from build123d import *

# Parameters (mm, degrees)
F1_DEPTH = 127
F2_R     = 242.677577
F3_DEPTH = 25.4
F4_R     = 14.944068
F5_DEPTH = 25.4
F6_DEPTH = 25.4
F7_DEPTH = 127.001


with BuildPart() as f1:
    # F0 (on Front) → F1 (new body)
    with BuildSketch(Plane.XZ):
        with BuildLine():
            Line((-211.768046, 98.819412), (-148.323849, 98.819412))
            Line((-148.323849, 98.819412), (-148.323849, -113.029018))
            ThreePointArc((-148.323849, -113.029018), (-234.634399, -80.514054), (-279.625744, 0))
            ThreePointArc((-279.625744, 0), (-245.041574, -121.948367), (-126.808003, -167.646199))
            ThreePointArc((-126.808003, -167.646199), (-8.574432, -121.948367), (26.009738, 0))
            ThreePointArc((26.009738, 0), (-18.981606, -80.514054), (-105.292156, -113.029018))
            Line((-105.292156, -113.029018), (-105.292156, 98.819412))
            Line((-105.292156, 98.819412), (-37.183784, 98.819412))
            Line((-37.183784, 98.819412), (-37.183784, 140.196055))
            Line((-37.183784, 140.196055), (-103.637077, 140.196055))
            Line((-103.637077, 140.196055), (-103.637077, 178.814262))
            Line((-103.637077, 178.814262), (-148.323849, 178.814262))
            Line((-148.323849, 178.814262), (-148.323849, 140.196055))
            Line((-148.323849, 140.196055), (-211.768046, 140.196055))
            Line((-211.768046, 140.196055), (-211.768046, 98.819412))
        make_face()
    extrude(amount=F1_DEPTH)

    # F2 (on Front) → F3 (join)
    with BuildSketch(Plane.XZ):
        with Locations((-129.646823, -14.895595)):
            Circle(F2_R)
    extrude(amount=F3_DEPTH)

    # F4 (on Front) → F5 (join)
    with BuildSketch(Plane.XZ):
        with Locations((-127.059489, 204.872638)):
            Circle(F4_R)
    extrude(amount=F5_DEPTH)

    # F4 (on Front) → F6 (join)
    with BuildSketch(Plane.XZ):
        with Locations((-127.059489, 204.872638)):
            Circle(F4_R)
    extrude(amount=F6_DEPTH)

    # F4 (on Front) → F7 (cut, through all)
    with BuildSketch(Plane.XZ):
        with Locations((-127.059489, 204.872638)):
            Circle(F4_R)
    extrude(amount=F7_DEPTH, mode=Mode.SUBTRACT)


solid = f1.part
Geometry: final body of the model. Coordinates: model frame, mm. A direction names the side the tool comes from. Round coordinates to 2 decimals unless told otherwise and drop trailing zeros. Loops run counter-clockwise (first coordinate to the right, second up) from the corner with the lowest first, then second, coordinate; pieces in that order, holes last.
Q1. Pin query (flat end, axial travel): P1, Ø1.5, axis at x = -227, y = -83, coming from the +Z side; P2, Ø11.5, axis at y = -58, z = 153, coming from the -X side; P3, Ø6, axis at x = -24.5, y = -92, coming from the -Z side. Return the tip coordinate at first contact, or that it passes through.
Q2. Access query for faces 1 (the flat face through (-126, -75, 178.814)), 2 (the cylindrical face through (-17.99, -75.49, -79.65)), 3 (the flat face through (-211.768, -75, 120)), 4 (the flat face through (-70, -75, 140.196)). Directions: +Z, -Z, +X, -X, +Y, -Y. A direction counts if a zero-diameter tool reaches every point of the face in a straight line with its end or side. Return the directions, or none.
Q3. Section A-A on z = 40. Return loops of the section in (x, y), plus the area to 3 significant figures.
Q4. Section B-B on x = -29.5. Return loops of the section in (y, z).
Q5. Material intervals for L1, parallel to X at y = -56, z = -83.5; L2, parallel to X at y = -113, z = -52; L3, parallel to X at y = -29, z = 22, sorted ascending.
Q6. Pull-direction query (X, two-part tool) for faces 5 (the cylindrical face through (-233.63, -75.49, -81.37)), 6 (the flat face through (-148.324, -75, -6)), 7 (the cylindrical face through (-182.255, -12.522, -251.802)), 8 (the flat face through (-180, -75, 140.196)); classes: released by +X, released by -X, zero draft, split by the parting line, or undercut.
Q7. Section C-C on y = -47.5. Return loops of the section in (x, z), plus the area to 3 significant figures.
Q8. Section D-D on y = -16.5. Return loops of the section in (x, z).
Evaluation:
1. P1: stops at z = -86.06
1. P2: stops at x = -148.32
1. P3: stops at z = -139.27
2. face 1: +Z, +X, -X, -Y
2. face 2: -Y
2. face 3: +Z, -X, -Y
2. face 4: +Z, +X, -Y
3. outline: (-366.03, -25.4) - (-148.32, -25.4) - (-148.32, -127) - (-105.29, -127) - (-105.29, -25.4) - (106.74, -25.4) - (106.74, 0) - (-366.03, 0) - close
3. area: 16,400 mm2
4. outline: (-127, -140.76) - (-25.4, -140.76) - (-25.4, -235.95) - (0, -235.95) - (0, 206.15) - (-25.4, 206.15) - (-25.4, -88.7) - (-127, -88.7) - close
5. L1: x = -270.06 to -231.04, -148.32 to -105.29, -22.57 to 16.44
5. L2: x = -279.74 to -259.57, -148.32 to -105.29, 5.95 to 26.13
5. L3: x = -148.32 to -105.29
6. face 5: undercut
6. face 6: undercut
6. face 7: split by the parting line
6. face 8: zero draft
7. outline: (-279.63, 0) arc R141.95 ccw to (-126.81, -167.65) arc R141.95 ccw to (26.01, 0) arc R134.32 cw to (-105.29, -113.03) - (-105.29, 98.82) - (-37.18, 98.82) - (-37.18, 140.2) - (-103.64, 140.2) - (-103.64, 178.81) - (-148.32, 178.81) - (-148.32, 140.2) - (-211.77, 140.2) - (-211.77, 98.82) - (-148.32, 98.82) - (-148.32, -113.03) arc R134.32 cw to start
7. area: 34,400 mm2
8. outline: circle Ø485.36 at (-129.65, -14.9); hole circle Ø29.89 at (-127.06, 204.87)
